Autodesk Inventor part; units mm, degrees
ref_plane "Work Plane1" through (6.35, 0, 0) normal (1, 0, 0) x (0, 1, 0)
ref_plane "YZ Plane" through (0, 0, 0) normal (1, 0, 0) x (0, 1, 0)
ref_plane "XZ Plane" through (0, 0, 0) normal (0, 1, 0) x (-1, 0, 0)
sketch "Sketch1" plane through (0, 0, 0) normal (0, 0, 1) x (1, 0, 0)
  circle A0 centre (0, 0) radius 6.35
  dimension "d0" = 12.7
extrude "Extrusion1" add sketch "Sketch1" along normal mid plane 127
sketch "Sketch2" plane through (0, 0, 63.5) normal (0, 0, 1) x (1, 0, 0)
  circle A0 centre (0, 0) radius 6.35
  line L0 (-4.5, 4.4802) -> (-4.5, -4.4802)
  line L1 (4.5, 4.4802) -> (4.5, -4.4802)
  line L2 (0, 0) -> (0, 6.1782) construction
  dimension "d3" = 9
extrude "Extrusion2" cut sketch "Sketch2" against normal blind 4 contours A0 L1 | L0 A0
sketch "Sketch3" plane through (0, 0, 63.5) normal (0, 0, 1) x (1, 0, 0)
  arc A0 (4.5, 4.4802) -> (-4.5, 4.4802) centre (0, 0) ccw
  circle A1 centre (0, 0) radius 3
  dimension "d6" = 6
extrude "Extrusion3" add sketch "Sketch3" along normal blind 8.2
chamfer "Chamfer1" distance 0.25 angle 45 4 edges at (-3, 0, 71.7) (0, -6.35, 63.5) (0, 6.35, 63.5) (-6.35, 0, -63.5)
ref_plane "Work Plane1" through (6.35, 0, 0) normal (1, 0, 0) x (0, 1, 0)
sketch "Sketch4" plane through (6.35, 0, 0) normal (1, 0, 0) x (0, 1, 0)
  line L0 (6.1, -63.5) -> (-6.1, -63.5)
  line L1 (0, -63.5) -> (0, -7.8695) construction
  line L2 (-1.5875, -63.5) -> (-1.5875, 30.1625)
  line L3 (0, 31.75) -> (0, 31.75)
  line L4 (1.5875, 30.1625) -> (1.5875, -63.5)
  arc A0 (0, 31.75) -> (-1.5875, 30.1625) centre (0, 30.1625) ccw
  arc A1 (1.5875, 30.1625) -> (0, 31.75) centre (0, 30.1625) ccw
  point P0 (1.5875, 31.75)
  dimension "d12" = 95.25
  dimension "d13" = 3.175
  dimension "d14" = 1.5875
extrude "Extrusion4" cut sketch "Sketch4" against normal blind 1.5875
sketch "Sketch5" plane through (0, 0, -63.5) normal (0, 0, -1) x (-1, 0, 0)
  arc A0 (-5.8898, -1.5875) -> (-5.8898, 1.5875) centre (0, 0) ccw
  circle A1 centre (0, 0) radius 4
  circle A2 centre (0, 0) radius 6.35
  dimension "d18" = 8
  dimension "d19" = 12.7
extrude "Extrusion5" cut sketch "Sketch5" against normal blind 12.7
chamfer "Chamfer2" distance 0.25 angle 45 3 edges at (4, 0, -63.5) (4, 0, -50.8) (-6.35, 0, -50.8)
properties part number "BB2-OutputShaft" material "Steel, Mild"
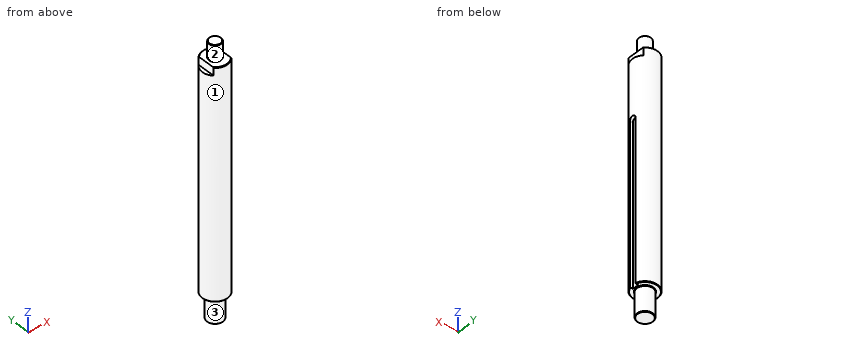
Input: part model. Units: mm. Frame: model coordinates. Face numbers are marked on the shaded views. A direction names the side the tool comes from. Give positions to 0.01 mm unless a question says otherwise; leave off trailing zeros. Order: outer loops, then holes, each group sorted by start corner. A loop starts at its lowest first (then second) coordinate and runs counter-clockwise, first axis right, second up. Notation, with made-up numbers: (84.5, 34) - (129.5, 34) arc R27 ccw to (129.5, 68) - close; hole circle Ø11 at (-5.75, 89). An arc over 180 degrees is marked (long way). Use a Markdown table: item, result.
(1) Pin query (flat end, axial travel): pin 1 (1.2 mm diameter, centred on y = 0.5, z = 62.5, fed in from +X); pin 2 (1 mm diameter, centred on y = 1.5, z = 35, fed in from +X); pin 3 (0.7 mm diameter, centred on x = 5.5, z = 0, fed in from -Y). Return the tip coordinate at first contact, or that it passes through.
Computed values:
| item | result |
|---|---|
| pin 1 | stops at x = 4.5 |
| pin 2 | stops at x = 6.27 |
| pin 3 | stops at y = -3.71 |
(2) Section query A-A (y = 0). Output: boundary loops of the cut face in (x, z), then the cut area to 3 significant figures.
Computed values:
| item | result |
|---|---|
| outline | (-6.35, -50.55) - (-6.1, -50.8) - (-4.25, -50.8) - (-4, -51.05) - (-4, -63.25) - (-3.75, -63.5) - (3.75, -63.5) - (4, -63.25) - (4, -51.05) - (4.25, -50.8) - (4.76, -50.8) - (4.76, 31.75) - (6.35, 31.75) - (6.35, 59.5) - (4.5, 59.5) - (4.5, 63.5) - (3, 63.5) - (3, 71.45) - (2.75, 71.7) - (-2.75, 71.7) - (-3, 71.45) - (-3, 63.5) - (-4.5, 63.5) - (-4.5, 59.5) - (-6.35, 59.5) - close |
| area | 1,460 mm2 |
(3) Access query for the marked faces 1, 2 and 3. Directions: +Z, -Z, +X, -X, +Y, -Y. A direction counts if a zero-diameter tool reaches every point of the face in a straight line with its end or side. Return the directions, or none.
Computed values:
| item | result |
|---|---|
| face 1 | +Z, -Z |
| face 2 | +Z |
| face 3 | -Z |
(4) Section query B-B (x = 0). Output: boundary loops of the cut face in (y, z).
Computed values:
| item | result |
|---|---|
| outline | (-6.35, -50.55) - (-6.1, -50.8) - (-4.25, -50.8) - (-4, -51.05) - (-4, -63.25) - (-3.75, -63.5) - (3.75, -63.5) - (4, -63.25) - (4, -51.05) - (4.25, -50.8) - (6.1, -50.8) - (6.35, -50.55) - (6.35, 63.25) - (6.1, 63.5) - (3, 63.5) - (3, 71.45) - (2.75, 71.7) - (-2.75, 71.7) - (-3, 71.45) - (-3, 63.5) - (-6.1, 63.5) - (-6.35, 63.25) - close |
(5) Section query C-C (z = -38). Output: boundary loops of the cut face in (x, y), then the cut area to 3 significant figures.
Computed values:
| item | result |
|---|---|
| outline | (4.76, -1.59) - (4.76, 1.59) - (6.15, 1.59) arc R6.35 ccw (long way) to (6.15, -1.59) - close |
| area | 122 mm2 |
(6) Line query: line 1 (Z direction, x = -5.25, y = -1.5); line 2 (Z direction, x = -0.75, y = -5); line 3 (Y direction, x = 0.5, z = -29.5). Output: solid intervals per line, ascending. Write a range as from..to.
Computed values:
| item | result |
|---|---|
| line 1 | z = -50.8..59.5 |
| line 2 | z = -50.8..63.5 |
| line 3 | y = -6.33..6.33 |
(7) Section query D-D (z = 36). Output: boundary loops of the cut face in (x, y).
Computed values:
| item | result |
|---|---|
| outline | circle Ø12.7 at (0, 0) |
